from build123d import *

# Parameters (mm, degrees)
SKETCH1_R           = 1.5
BOSS_EXTRUDE1_DEPTH = 6
BOSS_EXTRUDE2_DEPTH = 1
SKETCH4_R           = 1.5
CUT_EXTRUDE1_DEPTH  = 1


with BuildPart() as part:
    # Sketch1 → Boss-Extrude1 (new body)
    with BuildSketch(Plane(origin=(0, 0, 0), x_dir=(1, 0, 0), z_dir=(0, 1, 0))):
        Polygon((-6.890880132, -2.960704478), (-0.881394775, -7.448029488), (6.009485357, -4.48732501), (6.890880132, 2.960704478), (0.881394775, 7.448029488), (-6.009485357, 4.48732501), align=None)
        with Locations((2.445675843, -1.738841474)):
            Circle(SKETCH1_R, mode=Mode.SUBTRACT)
    extrude(amount=BOSS_EXTRUDE1_DEPTH)

    # Sketch2 → Boss-Extrude2 (add)
    with BuildSketch(Plane(origin=(0, 6, 0), x_dir=(1, 0, 0), z_dir=(0, 1, 0))):
        Polygon((8.269056159, 3.552845373), (1.05767373, 8.937635385), (-7.211382428, 5.384790012), (-8.269056159, -3.552845373), (-1.05767373, -8.937635385), (7.211382428, -5.384790012), align=None)
    extrude(amount=-BOSS_EXTRUDE2_DEPTH)

    # Sketch4 → Cut-Extrude1 (cut)
    with BuildSketch(Plane.XZ.offset(-5)):
        with Locations((2.445675843, 1.738841474)):
            Circle(SKETCH4_R)
    extrude(amount=-CUT_EXTRUDE1_DEPTH, mode=Mode.SUBTRACT)


solid = part.part
Can you work these out from the model? Positions are in its coordinate system, mm. A direction names the side the tool comes from. Round coordinates to 2 decimals unless told otherwise and drop trailing zeros. Loops run counter-clockwise (first coordinate to the right, second up) from the corner with the lowest first, then second, coordinate; pieces in that order, holes last. Notation, with made-up numbers: (76, 41.5) - (80, 41.5) arc R31 ccw to (80, 74.5) - close; hole circle Ø10 at (-0.75, -2.5). An arc over 180 degrees is marked (long way). Answer in a Markdown table with one row per item. Add a question column.
Q1. I want a section at A-A on z = 2.5. List the corners of the cut face in (x, y) for me.
Q2. Which directions (+Z, -Z, +X, -X, +Y, -Y) give clear straight access to the entire face, cutting with the end or side of a thin tool? Please do faces 1 (the flat face through (6.444, 2.465, 0.815)), 2 (the flat face through (-3, 5, -6)), 3 (the flat face through (3.93, 2.46, -5.17)).
Q3. I need wall thicknesses on L1, parallel to Z at x = 3.5, y = 4.6; L2, parallel to X at y = 2.25, z = 2.75; L3, parallel to X at y = 4.15, z = 3. Which ranges of each line are inside material? Lowest first, please.
Q4. I want a section at D-D on x = 0.25. List the corners of the cut face in (y, z) for me, and give its area (3 significant figures).
Q5. For pin 1 Ø1 at (x, y) = (-3, 4) entering from -Z; pin 2 Ø1 at (x, y) = (1, 3) entering from +Z; pin 3 Ø2 at (x, z) = (-5.5, -7) entering from -Y, each with a flat end and sliding along its axis, tell me the tip position at first contact or that it passes through.
Q6. I want a section at C-C on y = 5.4. List the corners of the cut face in (x, z) for me.
Q7. I want a section at B-B on x = 2.5. List the corners of the cut face in (y, z) for me.
A:
| question | item | result |
|---|---|---|
| 1 | outline | (-8.14, 5) - (-6.84, 5) - (-6.84, 0) - (1.15, 0) - (1.15, 6) - (-8.14, 6) - close; (3.74, 0) - (6.24, 0) - (6.24, 5) - (7.55, 5) - (7.55, 6) - (3.74, 6) - close |
| 2 | face 1 | +Z, +X, -Y |
| 2 | face 2 | -Y |
| 2 | face 3 | -Z, +X, -Y |
| 3 | L1 | -5.49 to 0.67, 2.81 to 5.57 |
| 3 | L2 | -6.87 to 1.34, 3.55 to 6.22 |
| 3 | L3 | -6.84 to 1.63, 3.26 to 6.19 |
| 4 | outline | (0, -7.18) - (5, -7.18) - (5, -8.59) - (6, -8.59) - (6, 8.38) - (5, 8.38) - (5, 6.96) - (0, 6.96) - close |
| 4 | area | 87.7 mm^2 |
| 5 | pin 1 | z = -6 |
| 5 | pin 2 | z = 6.85 |
| 5 | pin 3 | y = 5 |
| 6 | outline | (-8.27, 3.55) - (-7.21, -5.38) - (1.06, -8.94) - (8.27, -3.55) - (7.21, 5.38) - (-1.06, 8.94) - close; hole circle Ø3 at (2.45, 1.74) |
| 7 | outline | (0, -6.24) - (5, -6.24) - (5, -7.86) - (6, -7.86) - (6, 0.24) - (0, 0.24) - close; (0, 3.24) - (6, 3.24) - (6, 7.41) - (5, 7.41) - (5, 6) - (0, 6) - close |
